```python
from build123d import *

# Parameters (mm, degrees)
F1_DEPTH    = 44.958
F2_T1_DEPTH = 52.5754828874


# Not quite as in the source:
# - a fillet or chamfer that OpenCascade refuses, or shapes differently, is made with other operations: its cross-section is extruded or revolved along the edge and cut away or added


with BuildPart() as f1:
    # F0 (on Front) → F1 (new body)
    with BuildSketch(Plane.XZ):
        with BuildLine():
            Line((35.7939489186, 14.252791281), (-11.2892372768, 14.252791281))
            Line((-11.2892372768, 14.252791281), (-11.2892372768, -28.5055878506))
            Line((-11.2892372768, -28.5055878506), (20.2110526745, -28.5055878506))
            ThreePointArc((20.2110526745, -28.5055878506), (31.2298242792, -23.9414632112), (35.7939489186, -12.9226916064))
            Line((35.7939489186, -12.9226916064), (35.7939489186, 14.252791281))
        make_face()
    extrude(amount=F1_DEPTH)

    # F2: fillet of radius 5.08 on 1 edges, made by hand

    # F2_s2 → F2_t1 (cut)
    with BuildSketch(Plane.XY.offset(-25.6226916064)):
        with BuildLine():
            ThreePointArc((35.7939489186, -5.08), (34.306051367, -1.4878975516), (30.7139489186, 0))
            Line((30.7139489186, 0), (35.7939489186, 0))
            Line((35.7939489186, 0), (35.7939489186, -5.08))
        make_face()
    extrude(amount=F2_T1_DEPTH, mode=Mode.SUBTRACT)


solid = f1.part
```
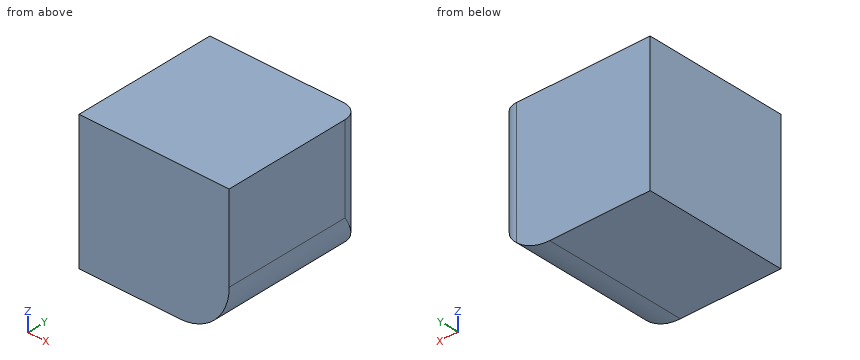
Part model, mm, in its own coordinate system. Round coordinates to 2 decimals unless told otherwise and drop trailing zeros. Loops run counter-clockwise (first coordinate to the right, second up) from the corner with the lowest first, then second, coordinate; pieces in that order, holes last.
Item 1: Cut at C-C, the plane x = 28. Give the cut face in (y, z).
Item 2: Cut at B-B, the plane z = -20. Give the cut face in (x, y).
Item 3: Drill centre lines: line 1 (X direction, y = -21.5, z = -18); line 2 (Z direction, x = 22, y = -26); line 3 (Y direction, x = 32, z = -6). Where is each one in solid material? Low to high.
Item 4: Drop a flat-ended pin along its axis: P1, Ø12, axis at y = -34, z = -22, coming from the +X side. Give the stop position or say it passes through.
Item 5: Cut at A-A, the plane y = -21. Give the cut face in (x, z), then the cut area to 3 significant figures.
A:
1. outline: (-44.96, -26.42) - (0, -26.42) - (0, 14.25) - (-44.96, 14.25) - close
2. outline: (-11.29, -44.96) - (34.09, -44.96) - (34.09, -1.29) arc R5.08 ccw to (30.71, 0) - (-11.29, 0) - close
3. line 1: x = -11.29 to 34.94
3. line 2: z = -28.4 to 14.25
3. line 3: y = -44.96 to -0.17
4. P1: stops at x = 35.49
5. outline: (-11.29, -28.51) - (20.21, -28.51) arc R15.58 ccw to (35.79, -12.92) - (35.79, 14.25) - (-11.29, 14.25) - close
5. area: 1,960 mm2
